Geometry: final body of the model. Coordinates: model frame, mm. Give positions to 0.01 mm unless a question says otherwise; leave off trailing zeros. Order: outer loops, then holes, each group sorted by start corner. A loop starts at its lowest first (then second) coordinate and runs counter-clockwise, first axis right, second up. Notation, with made-up numbers: (7, 38) -> (65, 38) arc R12 cw to (65, 51) -> close; hole circle Ø11 at (79, 10). An arc over 180 degrees is marked (long way). Answer in a Markdown table with one row per item. Add a question column.
Q1. Cut plane B-B on x = 9.5. Return the cut outline in (y, z), and give its area (3 significant figures).
Q2. Line query: line 1 along X through (y, z) = (0.8, 15.25); line 2 along X through (y, z) = (0.2, -2.5); line 3 along Z through (x, y) = (-9.5, 0.4). Output: solid intervals per line, ascending. Write a range as from..to.
Q3. Contact query for flat-ended pins moving along their axis: P1, Ø5, axis at x = -15.25, z = -15.25, coming from the -Y side; P2, Ø1, axis at x = -26.5, y = 1, coming from the -Z side; P3, Ø1, axis at x = -28.5, y = 0.5, coming from the +Z side. Output: stop coordinate, or through.
Q4. Cut plane C-C on y = 0.4. Return the cut outline in (x, z).
Q5. Cut plane D-D on z = 7.5. Return the cut outline in (x, y), and give its area (3 significant figures).
Q6. Cut plane A-A on z = -15.25. Return the cut outline in (x, y), and give its area (3 significant figures).
from build123d import *

# Parameters (mm, degrees)
CROQUIS1_W              = 16.5
CROQUIS1_H              = 17
CROQUIS1_R              = 1.5
CROQUIS1_W_2            = 5
SALIENTE_EXTRUIR1_DEPTH = 2


with BuildPart() as part:
    # Croquis1 → Saliente-Extruir1 (new body)
    # profile 1 of 3: a face of its own
    with BuildSketch(Plane(origin=(0, 0, 0), x_dir=(1, 0, 0), z_dir=(0, 1, 0))):
        with Locations((-26.25, 0)):
            Rectangle(CROQUIS1_W, CROQUIS1_H)
    # profile 2 of 3: a face of its own
    with BuildSketch(Plane(origin=(0, 0, 0), x_dir=(1, 0, 0), z_dir=(0, 1, 0))):
        Polygon((13, -13), (-13, -13), (-13, -8.5), (-18, -8.5), (-18, -18), (18, -18), (18, 18), (-18, 18), (-18, 8.5), (-13, 8.5), (-13, 13), (13, 13), align=None)
        with Locations(Location((-15.25, -15.25, 0), (0, 0, 270))):
            Circle(CROQUIS1_R, mode=Mode.SUBTRACT)
        with Locations(Location((15.25, -15.25, 0), (0, 0, 270))):
            Circle(CROQUIS1_R, mode=Mode.SUBTRACT)
        with Locations(Location((-15.25, 15.25, 0), (0, 0, 270))):
            Circle(CROQUIS1_R, mode=Mode.SUBTRACT)
        with Locations(Location((15.25, 15.25, 0), (0, 0, 270))):
            Circle(CROQUIS1_R, mode=Mode.SUBTRACT)
    # profile 3 of 3: a face of its own
    with BuildSketch(Plane(origin=(0, 0, 0), x_dir=(1, 0, 0), z_dir=(0, 1, 0))):
        with Locations((-15.5, 0)):
            Rectangle(CROQUIS1_W_2, CROQUIS1_H)
    extrude(amount=SALIENTE_EXTRUIR1_DEPTH)


solid = part.part
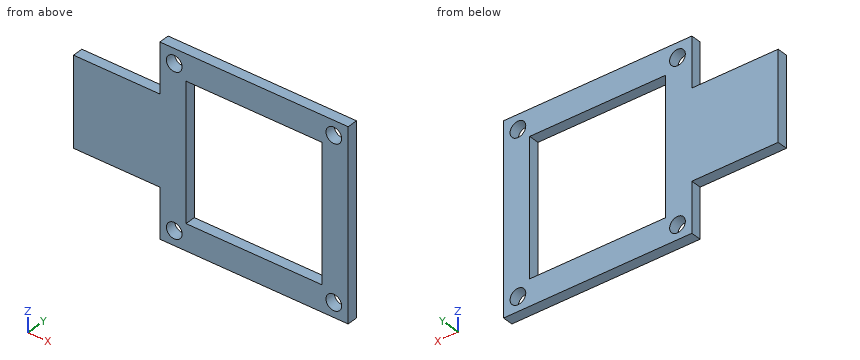
Completed:
| question | item | result |
|---|---|---|
| 1 | outline | (0, -18) -> (2, -18) -> (2, -13) -> (0, -13) -> close; (0, 13) -> (2, 13) -> (2, 18) -> (0, 18) -> close |
| 1 | area | 20.0 mm² |
| 2 | line 1 | x = -18..-16.75, -13.75..13.75, 16.75..18 |
| 2 | line 2 | x = -34.5..-13, 13..18 |
| 2 | line 3 | z = -18..-13, 13..18 |
| 3 | P1 | stops at y = 0 |
| 3 | P2 | stops at z = -8.5 |
| 3 | P3 | stops at z = 8.5 |
| 4 | outline | (-34.5, -8.5) -> (-18, -8.5) -> (-18, -18) -> (18, -18) -> (18, 18) -> (-18, 18) -> (-18, 8.5) -> (-34.5, 8.5) -> close; hole circle Ø3 at (-15.25, -15.25); hole circle Ø3 at (-15.25, 15.25); hole (-13, -13) -> (13, -13) -> (13, 13) -> (-13, 13) -> close; hole circle Ø3 at (15.25, -15.25); hole circle Ø3 at (15.25, 15.25) |
| 5 | outline | (-34.5, 0) -> (-13, 0) -> (-13, 2) -> (-34.5, 2) -> close; (13, 0) -> (18, 0) -> (18, 2) -> (13, 2) -> close |
| 5 | area | 53.0 mm² |
| 6 | outline | (-18, 0) -> (-16.75, 0) -> (-16.75, 2) -> (-18, 2) -> close; (-13.75, 0) -> (13.75, 0) -> (13.75, 2) -> (-13.75, 2) -> close; (16.75, 0) -> (18, 0) -> (18, 2) -> (16.75, 2) -> close |
| 6 | area | 60.0 mm² |
